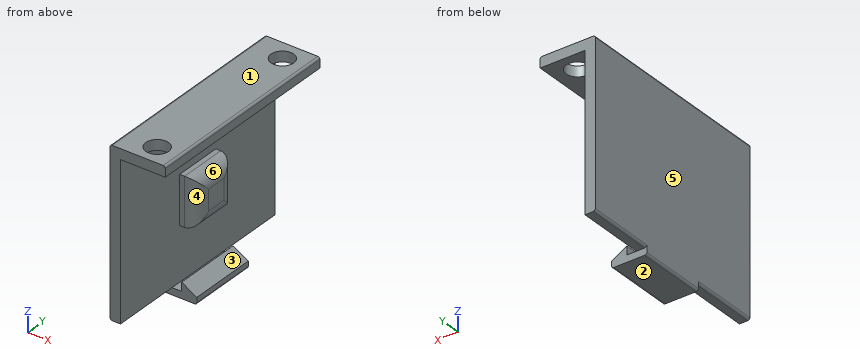
from build123d import *

# Parameters (mm, degrees)
BOSS_EXTRUDE1_DEPTH      = 5
BOSS_EXTRUDE1_DEPTH_BACK = 5
SKETCH2_W                = 3.6
SKETCH2_H                = 10
BOSS_EXTRUDE2_DEPTH      = 1
SKETCH3_W                = 1
SKETCH3_H                = 10
BOSS_EXTRUDE3_DEPTH      = 1.5
SKETCH4_W                = 1.5
SKETCH4_H                = 30
SKETCH4_W_2              = 6.5
SKETCH4_R                = 1.65
BOSS_EXTRUDE4_DEPTH      = 1.5
FILLET1_R                = 0.3
SKETCH5_W                = 7
SKETCH5_H                = 7
BOSS_EXTRUDE5_DEPTH      = 2.7
FILLET2_R                = 2


with BuildPart() as part:
    # Sketch1 → Boss-Extrude1 (new, two sides: drawn at the far end of the back side and taken through both)
    with BuildSketch(Plane(origin=(0, 0, 0), x_dir=(1, 0, 0), z_dir=(0, 1, 0)).offset(-BOSS_EXTRUDE1_DEPTH_BACK)):
        Polygon((0, 0), (-2.2, 0), (-2.2, -1.270170592), align=None)
    extrude(amount=BOSS_EXTRUDE1_DEPTH + BOSS_EXTRUDE1_DEPTH_BACK)

    # Sketch2 → Boss-Extrude2 (add)
    with BuildSketch(Plane(origin=(0, 0, 0), x_dir=(-1, 0, 0), z_dir=(0, 0, -1))):
        with Locations((1.8, 0)):
            Rectangle(SKETCH2_W, SKETCH2_H)
    extrude(amount=BOSS_EXTRUDE2_DEPTH)

    # Sketch3 → Boss-Extrude3 (add)
    with BuildSketch(Plane.ZY.offset(3.6)):
        Polygon((0, -5), (0, -15), (22.5, -15), (22.5, 15), (0, 15), (0, 5), align=None)
        with Locations((-0.5, 0)):
            Rectangle(SKETCH3_W, SKETCH3_H)
    extrude(amount=BOSS_EXTRUDE3_DEPTH)

    # Sketch4 → Boss-Extrude4 (add)
    # profile 1 of 2: a face of its own
    with BuildSketch(Plane.XY.offset(22.5)):
        with Locations((-4.35, 0)):
            Rectangle(SKETCH4_W, SKETCH4_H)
    # profile 2 of 2: a face of its own
    with BuildSketch(Plane.XY.offset(22.5)):
        with Locations((-0.35, 0)):
            Rectangle(SKETCH4_W_2, SKETCH4_H)
        with Locations((-0.4, -12.15)):
            Circle(SKETCH4_R, mode=Mode.SUBTRACT)
        with Locations((-0.4, 12.15)):
            Circle(SKETCH4_R, mode=Mode.SUBTRACT)
    extrude(amount=BOSS_EXTRUDE4_DEPTH)

    # Fillet1
    fillet1_edges = [part.edges().sort_by_distance(p)[0] for p in [
        (0, 0, -1),
        (-5.1, 10, 0),
        (-5.1, -10, 0),
        (-5.1, 0, -1),
        (2.9, 0, 24),
        (-5.1, 0, 24),
    ]]
    fillet(fillet1_edges, radius=FILLET1_R)

    # Sketch5 → Boss-Extrude5 (add)
    with BuildSketch(Plane(origin=(-3.6, 0, 0), x_dir=(0, 0, -1), z_dir=(1, 0, 0))):
        with Locations((-11.25, 0)):
            Rectangle(SKETCH5_W, SKETCH5_H)
    extrude(amount=BOSS_EXTRUDE5_DEPTH)

    # Fillet2
    fillet2_edges = [part.edges().sort_by_distance(p)[0] for p in [
        (-0.9, 0, 7.75),
        (-0.9, 3.5, 11.25),
        (-0.9, -3.5, 11.25),
        (-0.9, 0, 14.75),
    ]]
    fillet(fillet2_edges, radius=FILLET2_R)


solid = part.part
Source: CAD feature listing. Evaluate the final solid. Frame: model axes, mm. Face numbers are marked on the shaded views. A direction names the side the tool comes from. Give positions to 0.01 mm unless a question says otherwise; leave off trailing zeros. Write each loop counter-clockwise with the first axis right and the second up, starting at its lowest first coordinate (ties: lowest second). Pieces come first, ordered by that corner, then holes. Notation, with made-up numbers: M 53,89.5 L 69,89.5 A8 cw 69,94.5 Z; hole C 55.25,67.5 d6. An arc over 180 degrees is marked long. Return JSON: item names as keys, results as strings. Group by question number.
1) Set-up query: the marked faces 4, 5 and 6. Return all of +Z, -Z, +X, -X, +Y, -Y with unobstructed straight access to the full face (end or side cutting, diameter ignored); none if empty.
2) Pin query (flat end, axial travel): P1, Ø1.1, axis at x = -1.5, z = 0, coming from the +Y side; P2, Ø1.5, axis at y = -2, z = 11, coming from the +X side; P3, Ø1.1, axis at x = -2, z = 0.5, coming from the -Y side. Return the tip coordinate at first contact, or that it passes through.
3) Cut plane D-D, the plane z = 10.75. Output: boundary loops of the cut face in (x, y).
4) Cut plane A-A, the plane y = 12.15. Output: boundary loops of the cut face in (x, z), plus the area to 3 significant figures.
5) Cut plane C-C, the plane x = -1.5. Output: boundary loops of the cut face in (y, z).
6) Cut plane B-B, the plane y = -0.5. Output: boundary loops of the cut face in (x, z).
7) Pull-direction query (Z, two-part tool) for the marked faces 1, 2 and 3; classes: pulls with the +Z half, pulls with the -Z half, needs draft (parallel to the pull), parting line crosses it, or undercut.
8) Material intervals for line 1 along Y through (x, z) = (-0.4, 23.4); line 2 along Z through (x, y) = (-2.25, -9); line 3 along Z through (x, y) = (-2.5, 2.75), sorted ascending. Write a range as [from, to].
Recorded:
{
 "1": {"face 4": "+X, -Y", "face 5": "+Z, -Z, -X, +Y, -Y", "face 6": "+X, +Y, -Y"},
 "2": {"P1": "stops at y = 5", "P2": "stops at x = -0.9", "P3": "stops at y = -5"},
 "3": {"outline": "M -5.1,-15 L -3.6,-15 L -3.6,-3.5 L -2.9,-3.5 A2 ccw -0.9,-1.5 L -0.9,1.5 A2 ccw -2.9,3.5 L -3.6,3.5 L -3.6,15 L -5.1,15 Z"},
 "4": {"outline": "M -5.1,0.3 A0.3 ccw -4.8,0 L -3.6,0 L -3.6,22.5 L -2.05,22.5 L -2.05,24 L -4.8,24 A0.3 ccw -5.1,23.7 Z; M 1.25,22.5 L 2.9,22.5 L 2.9,23.7 A0.3 ccw 2.6,24 L 1.25,24 Z", "area": "40.7 mm²"},
 "5": {"outline": "M -15,22.5 L -13.38,22.5 L -13.38,24 L -15,24 Z; M -10.92,22.5 L 10.92,22.5 L 10.92,24 L -10.92,24 Z; M -5,-1 L 5,-1 L 5,0.87 L -5,0.87 Z; M -2.93,8.32 L 2.93,8.32 L 2.93,14.18 L -2.93,14.18 Z; M 13.38,22.5 L 15,22.5 L 15,24 L 13.38,24 Z"},
 "6": {"outline": "M -5.1,-0.7 A0.3 ccw -4.8,-1 L -0.3,-1 A0.3 ccw 0,-0.7 L 0,0 L -2.2,1.27 L -2.2,0 L -3.6,0 L -3.6,7.75 L -2.9,7.75 A2 ccw -0.9,9.75 L -0.9,12.75 A2 ccw -2.9,14.75 L -3.6,14.75 L -3.6,22.5 L 2.9,22.5 L 2.9,23.7 A0.3 ccw 2.6,24 L -4.8,24 A0.3 ccw -5.1,23.7 Z"},
 "7": {"face 1": "pulls with the +Z half", "face 2": "pulls with the -Z half", "face 3": "undercut"},
 "8": {"line 1": "y = [-15, -13.8], [-10.5, 10.5], [13.8, 15]", "line 2": "z = [22.5, 24]", "line 3": "z = [-1, 0], [7.79, 14.71], [22.5, 24]"}
}
